The listing builds one solid part. Answer for the finished solid, in the listing's coordinates (mm). Round coordinates to 2 decimals unless told otherwise and drop trailing zeros. Order: outer loops, then holes, each group sorted by start corner. A loop starts at its lowest first (then second) coordinate and runs counter-clockwise, first axis right, second up. Notation, with made-up numbers: (-7.75, -27) - (0.25, -27) arc R21 cw to (0.25, -7) - close; hole circle Ø9 at (15, 47.5). An arc over 180 degrees is marked (long way). Write item = value, one per line.
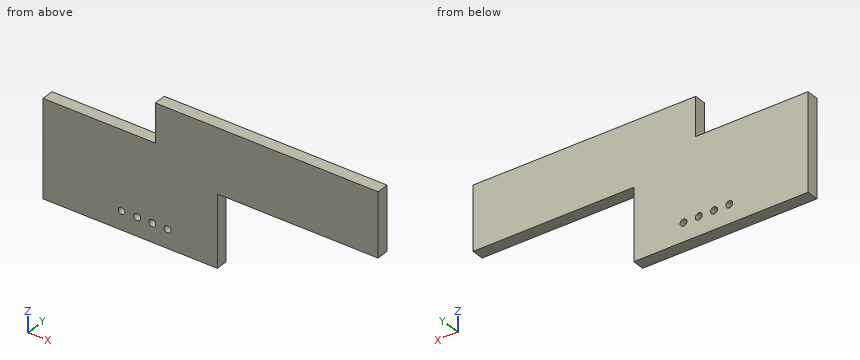
Autodesk Inventor part; units mm, degrees
ref_plane "YZ Plane" through (0, 0, 0) normal (1, 0, 0) x (0, 1, 0)
ref_plane "XZ Plane" through (0, 0, 0) normal (0, 1, 0) x (-1, 0, 0)
ref_plane "XY Plane" through (0, 0, 0) normal (0, 0, 1) x (1, 0, 0)
sketch "Sketch1" plane through (0, 0, 0) normal (0, 1, 0) x (-1, 0, 0)
  line L0 (-14.7409, 8.9608) -> (29.2011, 8.9608)
  line L1 (29.2011, 8.9608) -> (29.2011, -8.8192)
  line L2 (29.2011, -8.8192) -> (-14.7409, -8.8192)
  line L3 (-14.7409, -8.8192) -> (-14.7409, 8.9608)
  line L4 (-14.7409, 8.9608) -> (14.4691, 8.9608)
  line L5 (14.4691, 8.9608) -> (14.4691, 3.8808)
  line L6 (6.3411, 0.5788) -> (-14.7409, 0.5788)
  line L7 (-14.7409, 0.5788) -> (-14.7409, 8.9608)
  line L8 (29.2011, -8.8192) -> (6.3411, -8.8192)
  line L9 (6.3411, -8.8192) -> (6.3411, 0.5788)
  line L10 (14.4691, 3.8808) -> (29.2011, 3.8808)
  line L11 (29.2011, 3.8808) -> (29.2011, -8.8192)
  point P0 (0, 0)
  dimension "d0" = 43.942
  dimension "d1" = 17.78
  dimension "d2" = 21.082
  dimension "d3" = 14.732
  dimension "d4" = 9.398
  dimension "d5" = 5.08
extrude "Extrusion1" add sketch "Sketch1" along normal blind 1.6 contours L0 L5 L10 L1 L2 L9 L6 L3
sketch "Sketch2" plane through (0, 1.6, 0) normal (0, 1, 0) x (1, 0, 0)
  line L0 (-6.3411, -0.5788) -> (-6.3411, 8.8192)
  line L1 (-6.3411, 8.8192) -> (-29.2011, 8.8192)
  line L2 (-14.4691, -8.9608) -> (14.7409, -8.9608)
  circle A0 centre (-12.8689, 6.3808) radius 0.45
  line L3 (-18.8689, 6.3808) -> (-12.8689, 6.3808) construction
  circle A1 centre (-14.8689, 6.3808) radius 0.45
  circle A2 centre (-16.8689, 6.3808) radius 0.45
  circle A3 centre (-18.8689, 6.3808) radius 0.45
  point P0 (0, 0)
  dimension "d9" = 6.5278
  dimension "d15" = 0.9
  dimension "d16" = 2.4384
  dimension "d19" = 0.9
  dimension "d20" = 0.9
  dimension "d21" = 0.9
  dimension "d22" = 2
  dimension "d23" = 2
  dimension "d24" = 2
extrude "Extrusion2" cut sketch "Sketch2" against normal up to next
properties part number "MezzanineBoard"
Q1. Section C-C on x = -18 is taken. Determine the outline of the cut face in (y, z).
Model answer:
outline = (0, -8.82) - (1.6, -8.82) - (1.6, 3.88) - (0, 3.88) - close
Q2. Section A-A on y = 0.5 is taken. Determine the outline of the cut face in (x, z), then the cut area to 3 significant figures.
Model answer:
outline = (-29.2, -8.82) - (-6.34, -8.82) - (-6.34, 0.58) - (14.74, 0.58) - (14.74, 8.96) - (-14.47, 8.96) - (-14.47, 3.88) - (-29.2, 3.88) - close; hole circle Ø0.9 at (-18.87, -6.38); hole circle Ø0.9 at (-16.87, -6.38); hole circle Ø0.9 at (-14.87, -6.38); hole circle Ø0.9 at (-12.87, -6.38)
area = 506 mm^2
Q3. Find the intervals of material crossed by line 1 (X direction, y = 1.15, z = 6.75); line 2 (X direction, y = 0.1, z = -1.5); line 3 (Z direction, x = -19.5, y = 1.35), in increasing order. Write a range as from..to.
Model answer:
line_1 = -14.47..14.74
line_2 = -29.2..-6.34
line_3 = -8.82..3.88
Q4. Section B-B on z = -4 is taken. Determine the outline of the cut face in (x, y), then the cut area to 3 significant figures.
Model answer:
outline = (-29.2, 0) - (-6.34, 0) - (-6.34, 1.6) - (-29.2, 1.6) - close
area = 36.6 mm^2
